Input: part model. Units: mm. Frame: model coordinates. A direction names the side the tool comes from. Coordinates: 2 decimals unless noted, no trailing zeros. Write each loop counter-clockwise with the first axis right and the second up, starting at its lowest first coordinate (ties: lowest second). Pieces come first, ordered by that corner, then holes. Notation, with made-up numbers: (36.25, -32.5) - (49.25, -32.5) arc R20 cw to (49.25, -13.5) - close; hole circle Ø11 at (-20.75, 24.25). An arc over 180 degrees is marked (long way). Use a Markdown table: item, result. Add a question column.
Q1. Section query C-C (y = 3). Return the cut outline in (x, z), then the cut area to 3 significant figures.
Q2. Material intervals for probe 1 along Y at (x, z) = (37.5, 1.7); probe 2 along X at (y, z) = (3.75, 0.1); probe 3 along Y at (x, z) = (-13.5, 0.9), sorted ascending. Write a range as from..to.
Q3. Mould query, pull axis Y, two halves, no side actions, for faces 3 (the face through (41, 4.2, 1)), 4 (the face through (45, 0, 1)), 5 (the face through (-1.216, 1.115, 1.479)). Classes: released by +Y, released by -Y, zero draft, split by the parting line, or undercut.
Q4. Set-up query: faces 1 (the face through (-34.9, -0.84, 1.52)), 2 (the face through (-7, -1, 0)). Return all of +Z, -Z, +X, -X, +Y, -Y with unobstructed straight access to the full face (end or side cutting, diameter ignored); none if empty.
Q5. Section query D-D (x = -28). Return the cut outline in (y, z), then the cut area to 3 significant figures.
Q6. Pin query (flat end, axial travel): P1, Ø4, axis at x = 37.5, y = 0, coming from the +Z side; P2, Ø1, axis at y = -3, z = 1.5, coming from the -X side; P3, Ø1.5, axis at x = -13, z = 1, coming from the +Y side. Return the tip coordinate at first contact, or that it passes through.
Q7. Section query B-B (z = 1.5). Return the cut outline in (x, y), then the cut area to 3 significant figures.
Q8. Section query A-A (x = 0). Return the cut outline in (y, z), then the cut area to 3 significant figures.
from build123d import *

# Parameters (mm, degrees)
SKETCH1_R           = 1.65
BOSS_EXTRUDE1_DEPTH = 3
FILLET1_R           = 3


with BuildPart() as part:
    # Sketch1 → Boss-Extrude1 (new body)
    with BuildSketch(Plane.XY):
        with BuildLine():
            Line((-53.205266808, 1.8), (-46, 1.8))
            Line((-46, 1.8), (-46, -1.7))
            Line((-46, -1.7), (-34, -1.7))
            Line((-34, -1.7), (-34, 1.8))
            Line((-34, 1.8), (-3.794733192, 1.8))
            ThreePointArc((-3.794733192, 1.8), (0, 4.2), (3.794733192, 1.8))
            Line((3.794733192, 1.8), (33.705266808, 1.8))
            ThreePointArc((33.705266808, 1.8), (35.255005568, 3.54964787), (37.5, 4.2))
            Line((37.5, 4.2), (45, 4.2))
            Line((45, 4.2), (45, -4.2))
            Line((45, -4.2), (-57, -4.2))
            ThreePointArc((-57, -4.2), (-60.54964787, 2.244994432), (-53.205266808, 1.8))
        make_face()
        Circle(SKETCH1_R, mode=Mode.SUBTRACT)
        with Locations((-57, 0)):
            Circle(SKETCH1_R, mode=Mode.SUBTRACT)
        with Locations((37.5, 0)):
            Circle(SKETCH1_R, mode=Mode.SUBTRACT)
    extrude(amount=BOSS_EXTRUDE1_DEPTH)

    # Fillet1
    fillet1_edges = [part.edges().sort_by_distance(p)[0] for p in [
        (-46, -1.7, 1.5),
        (-34, -1.7, 1.5),
    ]]
    fillet(fillet1_edges, radius=FILLET1_R)


solid = part.part
Values follow:
| question | item | result |
|---|---|---|
| 1 | outline | (-59.94, 0) - (-54.06, 0) - (-54.06, 3) - (-59.94, 3) - close; (-2.94, 0) - (2.94, 0) - (2.94, 3) - (-2.94, 3) - close; (34.56, 0) - (45, 0) - (45, 3) - (34.56, 3) - close |
| 1 | area | 66.6 mm2 |
| 2 | probe 1 | -4.2..-1.65, 1.65..4.2 |
| 2 | probe 2 | -58.89..-55.11, -1.89..1.89, 35.61..45 |
| 2 | probe 3 | -4.2..1.8 |
| 3 | face 3 | released by +Y |
| 3 | face 4 | zero draft |
| 3 | face 5 | undercut |
| 4 | face 1 | +Z, -Z, +Y |
| 4 | face 2 | -Z, +X, -X, +Y, -Y |
| 5 | outline | (-4.2, 0) - (1.8, 0) - (1.8, 3) - (-4.2, 3) - close |
| 5 | area | 18.0 mm2 |
| 6 | P1 | z = 3 |
| 6 | P2 | x = -60.37 |
| 6 | P3 | y = 1.8 |
| 7 | outline | (-57, -4.2) - (45, -4.2) - (45, 4.2) - (37.5, 4.2) arc R4.2 ccw to (33.71, 1.8) - (3.79, 1.8) arc R4.2 ccw to (-3.79, 1.8) - (-34, 1.8) - (-34, 1.3) arc R3 cw to (-37, -1.7) - (-43, -1.7) arc R3 cw to (-46, 1.3) - (-46, 1.8) - (-53.21, 1.8) arc R4.2 ccw (long way) to start; hole circle Ø3.3 at (-57, 0); hole circle Ø3.3 at (0, 0); hole circle Ø3.3 at (37.5, 0) |
| 7 | area | 620 mm2 |
| 8 | outline | (-4.2, 0) - (-1.65, 0) - (-1.65, 3) - (-4.2, 3) - close; (1.65, 0) - (4.2, 0) - (4.2, 3) - (1.65, 3) - close |
| 8 | area | 15.3 mm2 |
